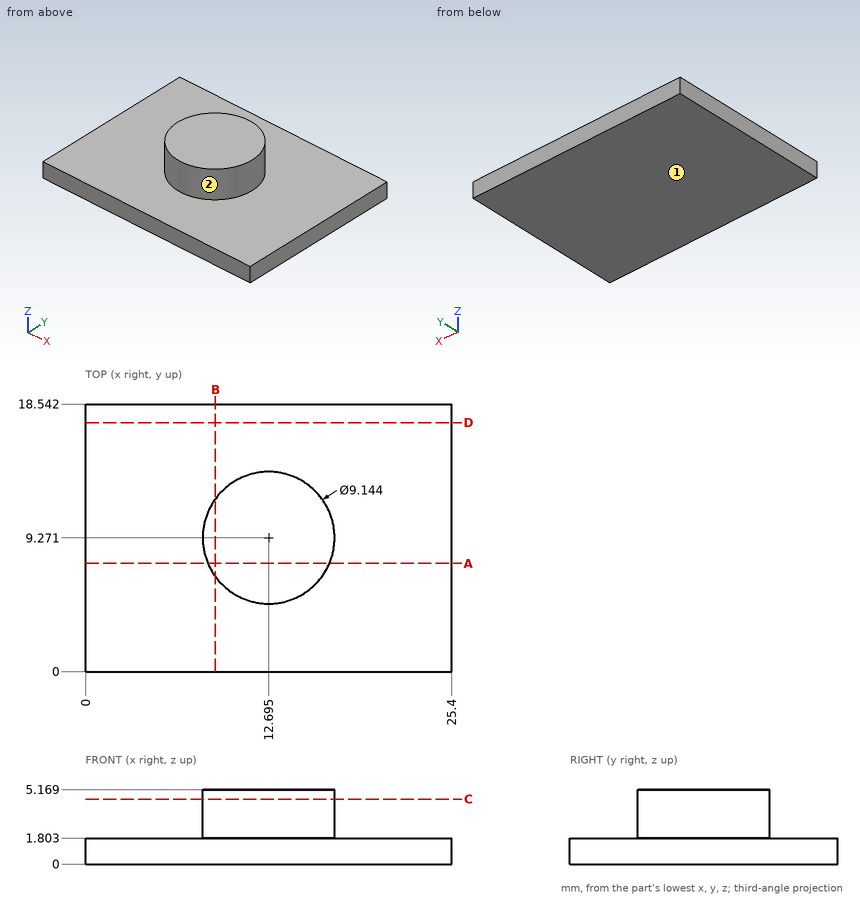
Input: dimensioned drawing with shaded views. Units: mm. Origin: part minimum x, y, z. A direction names the side the tool comes from. Give positions to 0.01 mm unless a question says otherwise; leave off trailing zeros. Write each loop counter-clockwise with the first axis right and the second up, starting at its lowest first coordinate (ties: lowest second). Pieces come first, ordered by that corner, then holes. Notation, with made-up numbers: (32, -27.75) -> (45, -27.75) arc R7 cw to (45, -21.75) -> close; hole circle Ø8 at (37, -2.75). An arc over 180 degrees is marked (long way). Answer as a JSON object with one key per item and string values.
1. Cut plane C-C on z = 4.5. Output: boundary loops of the cut face in (x, y) (1 decimal).
Ans:
{"outline": "circle Ø9.1 at (12.7, 9.3)"}
2. Ray query, probe 1 along Z at (x, y) = (7.5, 5.25); probe 2 along Y at (x, z) = (11.75, 1.85) (1 decimal); probe 3 along X at (y, z) = (10.25, 2.5). Return the intervals inside material, ascending. Write a range as from..to.
Ans:
{"probe 1": "z = 0..1.8", "probe 2": "y = 4.8..13.7", "probe 3": "x = 8.23..17.16"}
3. Access query for the marked faces 1 and 2. Directions: +Z, -Z, +X, -X, +Y, -Y. A direction counts if a zero-diameter tool reaches every point of the face in a straight line with its end or side. Return the directions, or none.
Ans:
{"face 1": "-Z, +X, -X, +Y, -Y", "face 2": "+Z"}
4. Cut plane D-D on y = 17.25. Output: boundary loops of the cut face in (x, z).
Ans:
{"outline": "(0, 0) -> (25.4, 0) -> (25.4, 1.8) -> (0, 1.8) -> close"}
5. Cut plane B-B on x = 9. Output: boundary loops of the cut face in (y, z).
Ans:
{"outline": "(0, 0) -> (18.54, 0) -> (18.54, 1.8) -> (11.96, 1.8) -> (11.96, 5.17) -> (6.58, 5.17) -> (6.58, 1.8) -> (0, 1.8) -> close"}
6. Cut plane A-A on y = 7.5. Output: boundary loops of the cut face in (x, z).
Ans:
{"outline": "(0, 0) -> (25.4, 0) -> (25.4, 1.8) -> (16.91, 1.8) -> (16.91, 5.17) -> (8.48, 5.17) -> (8.48, 1.8) -> (0, 1.8) -> close"}
